Geometry: see drawing. Coordinates: mm, zero at the bounding-box minimum. A direction names the side the tool comes from. Give positions to 0.01 mm unless a question says otherwise; leave off trailing zeros. Loops run counter-clockwise (first coordinate to the right, second up) from the corner with the lowest first, then second, coordinate; pieces in that order, holes last. Notation, with made-up numbers: (-34, -37) -> (5, -37) arc R24 ccw to (5, -10) -> close; hole circle Ø7 at (44.5, -25.5). An arc over 180 degrees is marked (long way). Return JSON: item names as keys, results as strings. Group by question number.
(1) Cut plane C-C on x = 14.25. Return loops of the section in (y, z) (1 decimal), then the cut area to 3 significant figures.
(2) Pin query (flat end, axial travel): pin 1 (1 mm diameter, centred on x = 14.29, y = 26.19, fed in from +Z) (3 decimals); pin 2 (1.5 mm diameter, centred on y = 15, z = 1.5, fed in from -X); pin 3 (2 mm diameter, centred on x = 10, z = 1.5, fed in from -Y); pin 4 (5 mm diameter, centred on x = 3, z = 4, fed in from -Y) (1 decimal). Return the tip coordinate at first contact, or that it passes through.
(3) Cut plane D-D on y = 19. Return loops of the section in (x, z) (1 decimal).
(4) Access query for the marked faces 5 and 6. Directions: +Z, -Z, +X, -X, +Y, -Y. A direction counts if a zero-diameter tool reaches every point of the face in a straight line with its end or side. Return the directions, or none.
(5) Cut plane B-B on y = 13.25. Return loops of the section in (x, z) (1 decimal), then the cut area to 3 significant figures.
(6) Ray query, line 1 (Z direction, x = 3, y = 9); line 2 (Y direction, x = 14, z = 2) (1 decimal); line 3 (X direction, y = 13, z = 9.75) (1 decimal). Return the intervals inside material, ascending. Write a range as from..to.
(7) Cut plane A-A on x = 2.5. Return loops of the section in (y, z).
(8) Draft query along Z for the marked faces 1, 2, 3 and 4. Return one class per face: released by +Z, released by -Z, zero draft, split by the parting line, or undercut.
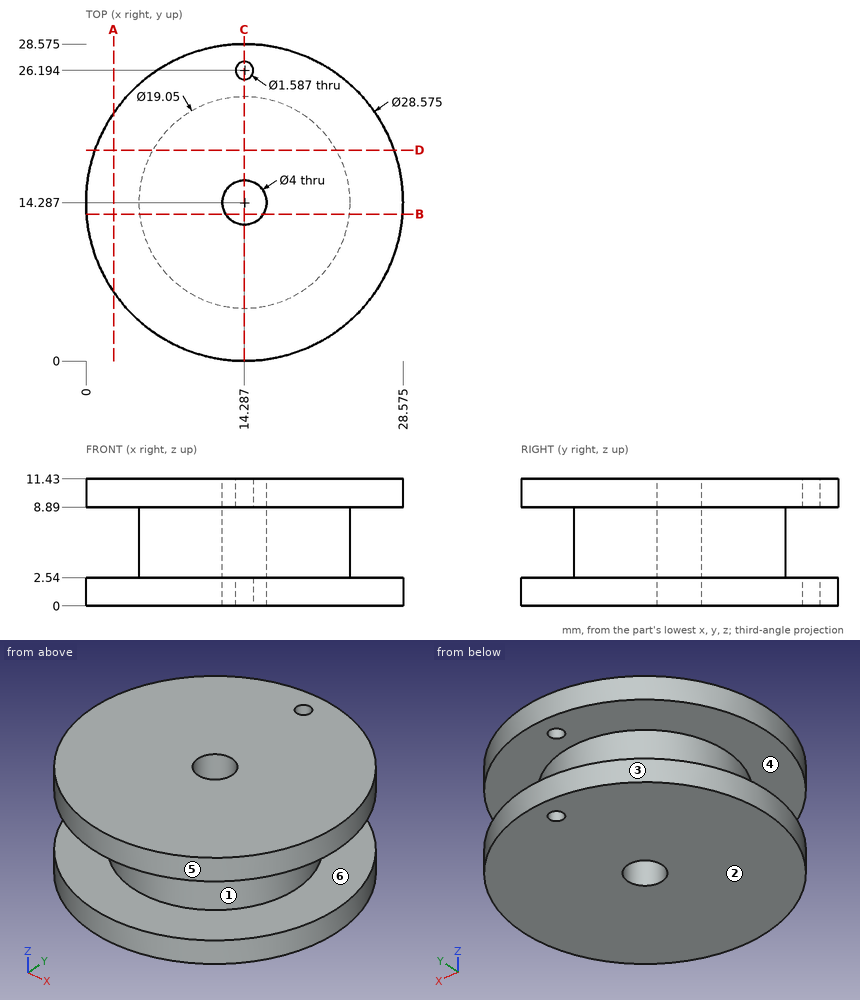
Answers:
{
 "1": {"outline": "(0, 0) -> (12.3, 0) -> (12.3, 11.4) -> (0, 11.4) -> (0, 8.9) -> (4.8, 8.9) -> (4.8, 2.5) -> (0, 2.5) -> close; (16.3, 0) -> (25.4, 0) -> (25.4, 2.5) -> (23.8, 2.5) -> (23.8, 8.9) -> (25.4, 8.9) -> (25.4, 11.4) -> (16.3, 11.4) -> close; (27, 0) -> (28.6, 0) -> (28.6, 2.5) -> (27, 2.5) -> close; (27, 8.9) -> (28.6, 8.9) -> (28.6, 11.4) -> (27, 11.4) -> close", "area": "212 mm²"},
 "2": {"pin 1": "through", "pin 2": "x = 0", "pin 3": "y = 0.38", "pin 4": "y = 3.4"},
 "3": {"outline": "(0.8, 0) -> (27.8, 0) -> (27.8, 2.5) -> (22.6, 2.5) -> (22.6, 8.9) -> (27.8, 8.9) -> (27.8, 11.4) -> (0.8, 11.4) -> (0.8, 8.9) -> (6, 8.9) -> (6, 2.5) -> (0.8, 2.5) -> close"},
 "4": {"face 5": "+Z, -Z", "face 6": "none"},
 "5": {"outline": "(0, 0) -> (12.6, 0) -> (12.6, 11.4) -> (0, 11.4) -> (0, 8.9) -> (4.8, 8.9) -> (4.8, 2.5) -> (0, 2.5) -> close; (16, 0) -> (28.5, 0) -> (28.5, 2.5) -> (23.8, 2.5) -> (23.8, 8.9) -> (28.5, 8.9) -> (28.5, 11.4) -> (16, 11.4) -> close", "area": "226 mm²"},
 "6": {"line 1": "0..2.54, 8.89..11.43", "line 2": "0..12.3, 16.3..25.5, 26.9..28.6", "line 3": "0.1..12.8, 15.8..28.5"},
 "7": {"outline": "(6.21, 0) -> (22.36, 0) -> (22.36, 2.54) -> (6.21, 2.54) -> close; (6.21, 8.89) -> (22.36, 8.89) -> (22.36, 11.43) -> (6.21, 11.43) -> close"},
 "8": {"face 1": "undercut", "face 2": "released by -Z", "face 3": "zero draft", "face 4": "undercut"}
}
